```python
from build123d import *

# Parameters (mm, degrees)
F0_R     = 2.1
F1_DEPTH = 60


with BuildPart() as f1:
    # F0 (on Top) → F1 (new body)
    with BuildSketch(Plane.XY):
        with BuildLine():
            Line((10, 4.410115), (10, 8.270115))
            ThreePointArc((10, 8.270115), (9.56066, 9.330775), (8.5, 9.770115))
            Line((8.5, 9.770115), (4.64, 9.770115))
            Line((4.64, 9.770115), (2.84, 7.970115))
            Line((2.84, 7.970115), (5.49934, 7.970115))
            Line((5.49934, 7.970115), (5.49934, 6.330115))
            Line((5.49934, 6.330115), (2.84, 3.670775))
            Line((2.84, 3.670775), (0.25, 3.670775))
            Line((0.25, 3.670775), (0, 3.420775))
            Line((0, 3.420775), (-0.25, 3.670775))
            Line((-0.25, 3.670775), (-2.84, 3.670775))
            Line((-2.84, 3.670775), (-5.49934, 6.330115))
            Line((-5.49934, 6.330115), (-5.49934, 7.970115))
            Line((-5.49934, 7.970115), (-2.84, 7.970115))
            Line((-2.84, 7.970115), (-4.64, 9.770115))
            Line((-4.64, 9.770115), (-8.5, 9.770115))
            ThreePointArc((-8.5, 9.770115), (-9.56066, 9.330775), (-10, 8.270115))
            Line((-10, 8.270115), (-10, 4.410115))
            Line((-10, 4.410115), (-8.2, 2.610115))
            Line((-8.2, 2.610115), (-8.2, 5.269455))
            Line((-8.2, 5.269455), (-6.56, 5.269455))
            Line((-6.56, 5.269455), (-3.90066, 2.610115))
            Line((-3.90066, 2.610115), (-3.90066, 0.020115))
            Line((-3.90066, 0.020115), (-3.65066, -0.229885))
            Line((-3.65066, -0.229885), (-3.90066, -0.479885))
            Line((-3.90066, -0.479885), (-3.90066, -3.069885))
            Line((-3.90066, -3.069885), (-6.56, -5.729225))
            Line((-6.56, -5.729225), (-8.2, -5.729225))
            Line((-8.2, -5.729225), (-8.2, -3.069885))
            Line((-8.2, -3.069885), (-10, -4.869885))
            Line((-10, -4.869885), (-10, -8.729885))
            ThreePointArc((-10, -8.729885), (-9.56066, -9.790545), (-8.5, -10.229885))
            Line((-8.5, -10.229885), (-4.64, -10.229885))
            Line((-4.64, -10.229885), (-2.84, -8.429885))
            Line((-2.84, -8.429885), (-5.49934, -8.429885))
            Line((-5.49934, -8.429885), (-5.49934, -6.789885))
            Line((-5.49934, -6.789885), (-2.84, -4.130545))
            Line((-2.84, -4.130545), (-0.25, -4.130545))
            Line((-0.25, -4.130545), (0, -3.880545))
            Line((0, -3.880545), (0.25, -4.130545))
            Line((0.25, -4.130545), (2.84, -4.130545))
            Line((2.84, -4.130545), (5.49934, -6.789885))
            Line((5.49934, -6.789885), (5.49934, -8.429885))
            Line((5.49934, -8.429885), (2.84, -8.429885))
            Line((2.84, -8.429885), (4.64, -10.229885))
            Line((4.64, -10.229885), (8.5, -10.229885))
            ThreePointArc((8.5, -10.229885), (9.56066, -9.790545), (10, -8.729885))
            Line((10, -8.729885), (10, -4.869885))
            Line((10, -4.869885), (8.2, -3.069885))
            Line((8.2, -3.069885), (8.2, -5.729225))
            Line((8.2, -5.729225), (6.56, -5.729225))
            Line((6.56, -5.729225), (3.90066, -3.069885))
            Line((3.90066, -3.069885), (3.90066, -0.479885))
            Line((3.90066, -0.479885), (3.65066, -0.229885))
            Line((3.65066, -0.229885), (3.90066, 0.020115))
            Line((3.90066, 0.020115), (3.90066, 2.610115))
            Line((3.90066, 2.610115), (6.56, 5.269455))
            Line((6.56, 5.269455), (8.2, 5.269455))
            Line((8.2, 5.269455), (8.2, 2.610115))
            Line((8.2, 2.610115), (10, 4.410115))
        make_face()
        Polygon((-6.56934, -7.859885), (-6.56934, -8.429885), (-8.2, -8.429885), (-8.2, -6.799225), (-7.63, -6.799225), align=None, mode=Mode.SUBTRACT)
        Polygon((8.2, -8.429885), (6.56934, -8.429885), (6.56934, -7.859885), (7.63, -6.799225), (8.2, -6.799225), align=None, mode=Mode.SUBTRACT)
        Polygon((-7.63, 6.339455), (-8.2, 6.339455), (-8.2, 7.970115), (-6.56934, 7.970115), (-6.56934, 7.400115), align=None, mode=Mode.SUBTRACT)
        with Locations((0, -0.229885)):
            Circle(F0_R, mode=Mode.SUBTRACT)
        Polygon((6.56934, 7.400115), (6.56934, 7.970115), (8.2, 7.970115), (8.2, 6.339455), (7.63, 6.339455), align=None, mode=Mode.SUBTRACT)
    extrude(amount=F1_DEPTH)


solid = f1.part
```
Can you work these out from the model? Positions are in its coordinate system, mm. A direction names the side the tool comes from. Coordinates: 2 decimals unless noted, no trailing zeros. Answer in a Markdown table with one row per item.
1. If I drill on line 1 along Y through (x, z) = (8, 9); line 2 along X through (y, z) = (-8, 5); line 3 along Y through (x, z) = (-7.25, 42.5), over which ranges is the centre line in solid material (lowest first)?
Reply:
| item | result |
|---|---|
| line 1 | y = -10.23 to -8.43, -6.8 to -5.73, 5.27 to 6.34, 7.97 to 9.77 |
| line 2 | x = -10 to -8.2, -6.57 to -5.5, 5.5 to 6.57, 8.2 to 10 |
| line 3 | y = -10.23 to -8.43, -7.18 to -5.73, 5.27 to 6.72, 7.97 to 9.77 |
2. For faces 1 (the flat face through (-3.75, -9.34, 29.58)), 2 (the flat face through (-2, 3.671, 30)), 3 (the flat face through (-4, 7.97, 30)), which set-ups out of +Z, -Z, +X, -X, +Y, -Y let a thin tool reach every point of the face, with its end or its side?
Reply:
| item | result |
|---|---|
| face 1 | +Z, -Z, -Y |
| face 2 | +Z, -Z, +Y |
| face 3 | +Z, -Z |
3. If we mould it in two halves opening along X, with no side actions, what happens to faces 4 (the flat face through (-4.15, 4.98, 29.58)), 5 (the flat face through (-9.09, -3.96, 29.58)), 6 (the flat face through (10, -7, 30))? For each: pulls with the +X half, pulls with the -X half, needs draft (parallel to the pull), parting line crosses it, or undercut.
Reply:
| item | result |
|---|---|
| face 4 | undercut |
| face 5 | pulls with the -X half |
| face 6 | pulls with the +X half |
4. For pin 1 (2 mm diameter, centred on y = -1, z = 16.5, fed in from -X); pin 2 (1.5 mm diameter, centred on x = -1.5, z = 9, fed in from -Y); pin 3 (0.8 mm diameter, centred on y = 1.5, z = 30, fed in from +X), each with a flat end and sliding along its axis, tell me the tip position at first contact or that it passes through.
Reply:
| item | result |
|---|---|
| pin 1 | stops at x = -3.9 |
| pin 2 | stops at y = -4.13 |
| pin 3 | stops at x = 3.9 |
5. Suppose I cut it at A-A (z = 42.5). Give the number of separate pieces and of enclosed holes in the cut face, and give its area (3 significant figures).
Reply:
| item | result |
|---|---|
| separate pieces | 1 |
| enclosed holes | 5 |
| area | 161 mm^2 |
